Build history of the part. All positions in model axes, mm. Round coordinates to 2 decimals unless told otherwise and drop trailing zeros. Order: outer loops, then holes, each group sorted by start corner. A loop starts at its lowest first (then second) coordinate and runs counter-clockwise, first axis right, second up. Notation, with made-up numbers: (-17, -11) -> (24, -11) arc R25 cw to (24, 26) -> close; hole circle Ø7 at (17.5, 83.5). An arc over 180 degrees is marked (long way). Answer as a JSON object with one key per item and string values.
from build123d import *

# Parameters (mm, degrees)
F1_DEPTH = 5


# Not quite as in the source:
# - a feature names something its author has since deleted; it is built from what else it names


with BuildPart() as f1:
    # F0 (on Front) → F1 (new body)
    with BuildSketch(Plane.XZ):
        with BuildLine():
            ThreePointArc((-6.5, 0), (-4.5961940777, 4.5961940777), (0, 6.5))
            Line((0, 6.5), (0, 10.16))
            ThreePointArc((0, 10.16), (-4.6323577324, 9.0425030738), (-8.2456907547, 5.9358389447))
            ThreePointArc((-8.2456907547, 5.9358389447), (-8.7368966018, 5.0442496049), (-9.2634326962, 4.173058193))
            ThreePointArc((-9.2634326962, 4.173058193), (-9.9333296581, 2.1341419594), (-10.16, 0))
            Line((-10.16, 0), (-6.5, 0))
        make_face()
        with BuildLine():
            ThreePointArc((-5.6291651246, -3.25), (-6.2785178709, -1.6823237932), (-6.5, 0))
            Line((-6.5, 0), (-10.16, 0))
            ThreePointArc((-10.16, 0), (-9.8138063951, -2.6296014982), (-8.7988181024, -5.08))
            Line((-8.7988181024, -5.08), (-5.6291651246, -3.25))
        make_face()
        with BuildLine():
            ThreePointArc((-1.0177419415, -10.1088971377), (-0.508973166, -10.0935992038), (0, -10.0884992098))
            Line((0, -10.0884992098), (0, -6.5))
            ThreePointArc((0, -6.5), (-3.25, -5.6291651246), (-5.6291651246, -3.25))
            Line((-5.6291651246, -3.25), (-8.7988181024, -5.08))
            ThreePointArc((-8.7988181024, -5.08), (-5.5148585095, -8.5329910126), (-1.0177419415, -10.1088971377))
        make_face()
        with BuildLine():
            ThreePointArc((1.0177419415, -10.1088971377), (5.5148585095, -8.5329910126), (8.7988181024, -5.08))
            Line((8.7988181024, -5.08), (5.6291651246, -3.25))
            ThreePointArc((5.6291651246, -3.25), (3.25, -5.6291651246), (0, -6.5))
            Line((0, -6.5), (0, -10.0884992098))
            ThreePointArc((0, -10.0884992098), (0.508973166, -10.0935992038), (1.0177419415, -10.1088971377))
        make_face()
        with BuildLine():
            ThreePointArc((8.7988181024, -5.08), (9.8138063951, -2.6296014982), (10.16, 0))
            Line((10.16, 0), (6.5, 0))
            ThreePointArc((6.5, 0), (6.2785178709, -1.6823237932), (5.6291651246, -3.25))
            Line((5.6291651246, -3.25), (8.7988181024, -5.08))
        make_face()
        with BuildLine():
            Line((6.5, 0), (10.16, 0))
            ThreePointArc((10.16, 0), (9.9333296581, 2.1341419594), (9.2634326962, 4.173058193))
            ThreePointArc((9.2634326962, 4.173058193), (8.7368966018, 5.0442496049), (8.2456907547, 5.9358389447))
            ThreePointArc((8.2456907547, 5.9358389447), (4.6323577324, 9.0425030738), (0, 10.16))
            Line((0, 10.16), (0, 6.5))
            ThreePointArc((0, 6.5), (4.5961940777, 4.5961940777), (6.5, 0))
        make_face()
        with BuildLine():
            ThreePointArc((-8.2456907547, 5.9358389447), (-4.6323577324, 9.0425030738), (0, 10.16))
            Line((0, 10.16), (0, 15.875))
            Line((0, 15.875), (0, 17.4625))
            ThreePointArc((0, 17.4625), (-3.175, 18.313238686), (-5.499261314, 20.6375))
            ThreePointArc((-5.499261314, 20.6375), (-5.7658770412, 13.0799448007), (-8.2456907547, 5.9358389447))
        make_face()
        with BuildLine():
            Line((-5.499261314, 20.6375), (0, 23.8125))
            Line((0, 23.8125), (0, 30.1625))
            ThreePointArc((0, 30.1625), (-5.499261314, 26.9875), (-5.499261314, 20.6375))
        make_face()
        with BuildLine():
            Line((0, 23.8125), (5.499261314, 20.6375))
            ThreePointArc((5.499261314, 20.6375), (6.1336289969, 22.1689990636), (6.35, 23.8125))
            ThreePointArc((6.35, 23.8125), (4.4901280605, 28.3026280605), (0, 30.1625))
            Line((0, 30.1625), (0, 23.8125))
        make_face()
        with BuildLine():
            ThreePointArc((0, 17.4625), (3.175, 18.313238686), (5.499261314, 20.6375))
            Line((5.499261314, 20.6375), (0, 23.8125))
            Line((0, 23.8125), (0, 17.4625))
        make_face()
        with BuildLine():
            ThreePointArc((-5.499261314, 20.6375), (-3.175, 18.313238686), (0, 17.4625))
            Line((0, 17.4625), (0, 23.8125))
            Line((0, 23.8125), (-5.499261314, 20.6375))
        make_face()
        with BuildLine():
            Line((-20.6222299276, -5.55625), (-20.6222299276, -11.90625))
            Line((-20.6222299276, -11.90625), (-15.1229686136, -8.73125))
            ThreePointArc((-15.1229686136, -8.73125), (-17.4472299276, -6.406988686), (-20.6222299276, -5.55625))
        make_face()
        with BuildLine():
            Line((-23.7972299276, -6.406988686), (-20.6222299276, -11.90625))
            Line((-20.6222299276, -11.90625), (-20.6222299276, -5.55625))
            ThreePointArc((-20.6222299276, -5.55625), (-22.265730864, -5.7726210031), (-23.7972299276, -6.406988686))
        make_face()
        with BuildLine():
            ThreePointArc((-23.7972299276, -6.406988686), (-26.7558589246, -10.2627490636), (-26.1214912416, -15.08125))
            Line((-26.1214912416, -15.08125), (-20.6222299276, -11.90625))
            Line((-20.6222299276, -11.90625), (-23.7972299276, -6.406988686))
        make_face()
        with BuildLine():
            ThreePointArc((-26.1214912416, -15.08125), (-20.6222299276, -18.25625), (-15.1229686136, -15.08125))
            Line((-15.1229686136, -15.08125), (-20.6222299276, -11.90625))
            Line((-20.6222299276, -11.90625), (-26.1214912416, -15.08125))
        make_face()
        with BuildLine():
            Line((-20.6222299276, -11.90625), (-15.1229686136, -15.08125))
            ThreePointArc((-15.1229686136, -15.08125), (-14.4886009307, -13.5497509364), (-14.2722299276, -11.90625))
            ThreePointArc((-14.2722299276, -11.90625), (-14.4886009307, -10.2627490636), (-15.1229686136, -8.73125))
            Line((-15.1229686136, -8.73125), (-20.6222299276, -11.90625))
        make_face()
        with BuildLine():
            Line((20.6222299276, -11.90625), (15.1229686136, -15.08125))
            ThreePointArc((15.1229686136, -15.08125), (20.6222299276, -18.25625), (26.1214912416, -15.08125))
            Line((26.1214912416, -15.08125), (20.6222299276, -11.90625))
        make_face()
        with BuildLine():
            ThreePointArc((26.9722299276, -11.90625), (25.1123579882, -7.4161219395), (20.6222299276, -5.55625))
            Line((20.6222299276, -5.55625), (20.6222299276, -11.90625))
            Line((20.6222299276, -11.90625), (26.1214912416, -15.08125))
            ThreePointArc((26.1214912416, -15.08125), (26.7558589246, -13.5497509364), (26.9722299276, -11.90625))
        make_face()
        with BuildLine():
            Line((20.6222299276, -11.90625), (20.6222299276, -5.55625))
            ThreePointArc((20.6222299276, -5.55625), (17.4472299276, -6.406988686), (15.1229686136, -8.73125))
            Line((15.1229686136, -8.73125), (20.6222299276, -11.90625))
        make_face()
        with BuildLine():
            ThreePointArc((15.1229686136, -8.73125), (14.2722299276, -11.90625), (15.1229686136, -15.08125))
            Line((15.1229686136, -15.08125), (20.6222299276, -11.90625))
            Line((20.6222299276, -11.90625), (15.1229686136, -8.73125))
        make_face()
        with BuildLine():
            ThreePointArc((-15.1229686136, -15.08125), (-8.4446259569, -11.5333683931), (-1.0177419415, -10.1088971377))
            ThreePointArc((-1.0177419415, -10.1088971377), (-5.5148585095, -8.5329910126), (-8.7988181024, -5.08))
            Line((-8.7988181024, -5.08), (-13.7481532851, -7.9375))
            Line((-13.7481532851, -7.9375), (-15.1229686136, -8.73125))
            ThreePointArc((-15.1229686136, -8.73125), (-14.4886009307, -10.2627490636), (-14.2722299276, -11.90625))
            ThreePointArc((-14.2722299276, -11.90625), (-14.4886009307, -13.5497509364), (-15.1229686136, -15.08125))
        make_face()
        with BuildLine():
            ThreePointArc((0, 10.16), (4.6323577324, 9.0425030738), (8.2456907547, 5.9358389447))
            ThreePointArc((8.2456907547, 5.9358389447), (5.7658770412, 13.0799448007), (5.499261314, 20.6375))
            ThreePointArc((5.499261314, 20.6375), (3.175, 18.313238686), (0, 17.4625))
            Line((0, 17.4625), (0, 15.875))
            Line((0, 15.875), (0, 10.16))
        make_face()
        with BuildLine():
            Line((12.5597401985, 0), (10.16, 0))
            ThreePointArc((10.16, 0), (9.8138063951, -2.6296014982), (8.7988181024, -5.08))
            Line((8.7988181024, -5.08), (13.7481532851, -7.9375))
            Line((13.7481532851, -7.9375), (15.1229686136, -8.73125))
            ThreePointArc((15.1229686136, -8.73125), (17.4472299276, -6.406988686), (20.6222299276, -5.55625))
            ThreePointArc((20.6222299276, -5.55625), (16.3207116364, -3.1703097876), (12.5597401985, 0))
        make_face()
        with BuildLine():
            ThreePointArc((-8.7988181024, -5.08), (-9.8138063951, -2.6296014982), (-10.16, 0))
            Line((-10.16, 0), (-12.5597401985, 0))
            ThreePointArc((-12.5597401985, 0), (-16.3207116364, -3.1703097876), (-20.6222299276, -5.55625))
            ThreePointArc((-20.6222299276, -5.55625), (-17.4472299276, -6.406988686), (-15.1229686136, -8.73125))
            Line((-15.1229686136, -8.73125), (-13.7481532851, -7.9375))
            Line((-13.7481532851, -7.9375), (-8.7988181024, -5.08))
        make_face()
        with BuildLine():
            Line((13.7481532851, -7.9375), (8.7988181024, -5.08))
            ThreePointArc((8.7988181024, -5.08), (5.5148585095, -8.5329910126), (1.0177419415, -10.1088971377))
            ThreePointArc((1.0177419415, -10.1088971377), (8.4446259569, -11.5333683931), (15.1229686136, -15.08125))
            ThreePointArc((15.1229686136, -15.08125), (14.2722299276, -11.90625), (15.1229686136, -8.73125))
            Line((15.1229686136, -8.73125), (13.7481532851, -7.9375))
        make_face()
        with BuildLine():
            Line((-12.5597401985, 0), (-10.16, 0))
            ThreePointArc((-10.16, 0), (-9.9333296581, 2.1341419594), (-9.2634326962, 4.173058193))
            ThreePointArc((-9.2634326962, 4.173058193), (-10.8020734635, 2.0000245587), (-12.5597401985, 0))
        make_face()
        with BuildLine():
            ThreePointArc((9.2634326962, 4.173058193), (9.9333296581, 2.1341419594), (10.16, 0))
            Line((10.16, 0), (12.5597401985, 0))
            ThreePointArc((12.5597401985, 0), (10.8020734635, 2.0000245587), (9.2634326962, 4.173058193))
        make_face()
    extrude(amount=F1_DEPTH)


solid = f1.part
1) Cut at B-B, the plane x = 4.5. Give the cut face in (y, z).
Checked values:
{"outline": "(-5, -10.49) -> (0, -10.49) -> (0, -4.69) -> (-5, -4.69) -> close; (-5, 4.69) -> (0, 4.69) -> (0, 28.29) -> (-5, 28.29) -> close"}
2) Flat gauge pins, fed straight in: pin 1 Ø3 at (x, y) = (18, -1.5) entering from -Z; pin 2 Ø1 at (y, z) = (-2, 5) entering from +X; pin 3 Ø1.5 at (y, z) = (-1.5, 3.5) entering from -X. Where does each tip first touch, or does it go through?
Checked values:
{"pin 1": "stops at z = -18.16", "pin 2": "stops at x = 9.06", "pin 3": "stops at x = -10.23"}
3) Cut at A-A, the plane z = 2. Give the cut face in (x, y), plus the area to 3 significant figures.
Checked values:
{"outline": "(-10.8, -5) -> (-6.18, -5) -> (-6.18, 0) -> (-10.8, 0) -> close; (6.18, -5) -> (10.8, -5) -> (10.8, 0) -> (6.18, 0) -> close", "area": "46.2 mm²"}
4) Cut at C-C, the plane y = -1.5. Give the cut face in (x, z), plus the area to 3 significant figures.
Checked values:
{"outline": "(-20.62, -5.56) arc R6.35 ccw (long way) to (-15.12, -15.08) arc R25.4 cw to (15.12, -15.08) arc R6.35 ccw (long way) to (20.62, -5.56) arc R25.4 cw to (5.5, 20.64) arc R6.35 ccw (long way) to (-5.5, 20.64) arc R25.4 cw to start; hole circle Ø13 at (0, 0)", "area": "889 mm²"}
5) Probe L1, parallel to Z at x = -2.5, y = -3; L2, parallel to X at y = -2.1, z = -2; L3, parallel to X at y = -4.4, z = -13.5. List the from-to ranges inside material, lowest first. Write a range as from..to.
Checked values:
{"L1": "z = -10.21..-6, 6..29.65", "L2": "x = -14.76..-6.18, 6.18..14.76", "L3": "x = -26.77..-12.71, 12.71..26.77"}
6) Cut at D-D, the plane z = -8. Give the cut face in (x, y).
Checked values:
{"outline": "(-25.63, -5) -> (25.63, -5) -> (25.63, 0) -> (-25.63, 0) -> close"}
